The drawing under review shows one solid part. Ordinate dimensions are in mm from its lowest x, y, z. A direction names the side the tool comes from. Round coordinates to 2 decimals unless told otherwise and drop trailing zeros. Order: outer loops, then holes, each group sorted by start corner. A loop starts at its lowest first (then second) coordinate and runs counter-clockwise, first axis right, second up. Notation, with made-up numbers: M -2.75,-1 L 3.25,-1 A20 ccw 3.25,25 Z; hole C -23,-32 d2. An arc over 180 degrees is marked long. Answer as a JSON object with one key per item and string values. Group by question number.
1) Consider section A-A, the plane y = 11. Write out the cut boundary in (x, z), then the cut area to 4 significant figures.
2) To check wall thickness, follow line 1 (X direction, y = 18.5, z = 16.25); line 2 (Z direction, x = 7.5, y = 10.5); line 3 (Z direction, x = 1.75, y = 20.5). State the ranges of each line that lie inside material, in increasing order.
3) Consider section D-D, the plane x = 24.5. Write out the cut boundary in (y, z), then the cut area to 3 significant figures.
4) Consider section C-C, the plane x = 5.5. Write out the cut boundary in (y, z), then the cut area to 3 significant figures.
5) For the marked faces 1 and 2, list the 3-axis set-ups (+Z, -Z, +X, -X, +Y, -Y) from which the entire face can be reached by the end or side of a thin tool; tool diameter is ignored.
6) Insertion check: pin 1 Ø5 at (x, z) = (22.5, 9.5) entering from +Y; pin 2 Ø12 at (y, z) = (15.5, 3) entering from -X; pin 3 Ø8 at (x, y) = (14.5, 4) entering from +Z; pin 4 Ø8 at (y, z) = (11.5, 19) entering from +X. Each pin has a flat end and moves straight along its axis. Give the tip position at first contact, or say it passes through.
7) The part is to be moulded in two halves that separate along Y. For the marked faces 3 and 4, say which applies: +Y half, -Y half, draft (parallel to the pull), parting line (faces both ways), or undercut.
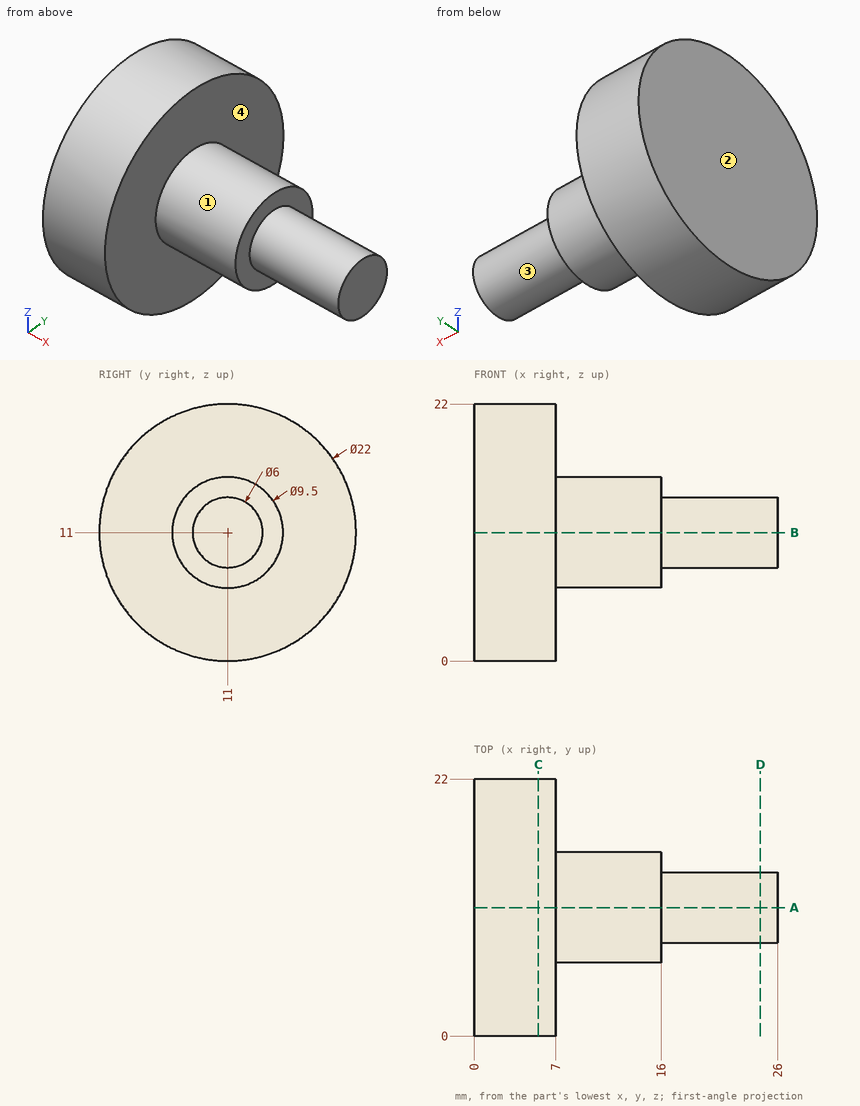
Results list:
{
 "1": {"outline": "M 0,0 L 7,0 L 7,6.25 L 16,6.25 L 16,8 L 26,8 L 26,14 L 16,14 L 16,15.75 L 7,15.75 L 7,22 L 0,22 Z", "area": "299.5 mm^2"},
 "2": {"line 1": "0 to 7", "line 2": "6.28 to 15.72", "line 3": "5.45 to 16.55"},
 "3": {"outline": "C 11,11 d6", "area": "28.3 mm^2"},
 "4": {"outline": "C 11,11 d22", "area": "380 mm^2"},
 "5": {"face 1": "+X", "face 2": "+Z, -Z, -X, +Y, -Y"},
 "6": {"pin 1": "y = 14", "pin 2": "x = 0", "pin 3": "z = 14.68", "pin 4": "x = 16"},
 "7": {"face 3": "parting line", "face 4": "draft"}
}
